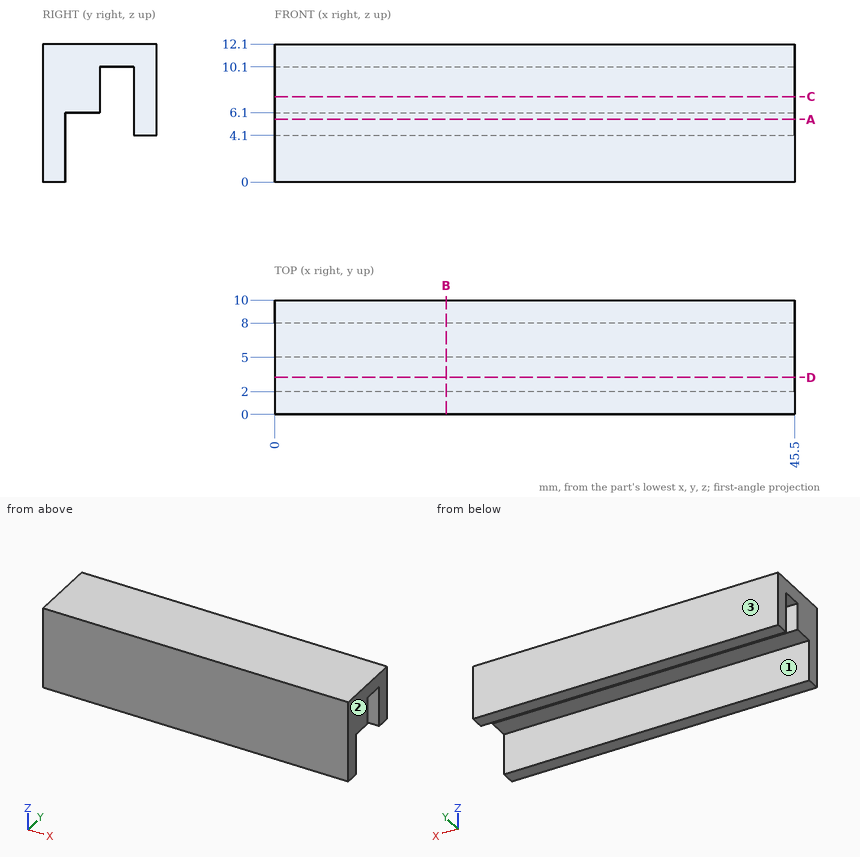
Geometry check sheet. Reference: drawing and pictorial views, mm from the part's lowest x, y, z. Coordinates: 2 decimals unless noted, no trailing zeros. Write each loop counter-clockwise with the first axis right and the second up, starting at its lowest first coordinate (ties: lowest second). Pieces come first, ordered by that corner, then holes. Notation, with made-up numbers: M -14,34.5 L 10,34.5 A14 ccw 10,59.5 Z; hole C 78.5,54.5 d6. An arc over 180 degrees is marked long. One line per question, with ' | ' between items.
1) Sectioned sample at A-A on z = 5.5. Record the cut outline in (x, y).
Solutions:
outline: M 0,0 L 45.5,0 L 45.5,2 L 0,2 Z; M 0,8 L 45.5,8 L 45.5,10 L 0,10 Z
2) Release check for a two-part mould opening along Y. For the marked faces 1, 2 and 3 record: +Y half, -Y half, draft (parallel to the pull), parting line (faces both ways), or undercut.
Solutions:
face 1: undercut | face 2: draft | face 3: +Y half
3) Sectioned sample at D-D on y = 3.25. Record the cut outline in (x, z), then the cut area to 3 significant figures.
Solutions:
outline: M 0,6.1 L 45.5,6.1 L 45.5,12.1 L 0,12.1 Z | area: 273 mm^2
4) Depth check by flat-ended pin: pin 1 Ø5 at (x, y) = (12.5, 7) entering from -Z; pin 2 Ø2 at (x, z) = (39, 2) entering from +Y; pin 3 Ø2.5 at (x, y) = (18.5, 6) entering from -Z. Enter the tip coordinate at first touch or a pass-through.
Solutions:
pin 1: z = 4.1 | pin 2: y = 2 | pin 3: z = 6.1
5) Sectioned sample at B-B on x = 15. Record the cut outline in (y, z).
Solutions:
outline: M 0,0 L 2,0 L 2,6.1 L 5,6.1 L 5,10.1 L 8,10.1 L 8,4.1 L 10,4.1 L 10,12.1 L 0,12.1 Z
6) Material ranges on L1, parallel to Y at x = 19, z = 8.5; L2, parallel to Y at x = 15, z = 6; L3, parallel to Z at x = 35.5, y = 3.25, recorded low to high.
Solutions:
L1: 0 to 5, 8 to 10 | L2: 0 to 2, 8 to 10 | L3: 6.1 to 12.1
7) Sectioned sample at C-C on z = 7.5. Record the cut outline in (x, y).
Solutions:
outline: M 0,0 L 45.5,0 L 45.5,5 L 0,5 Z; M 0,8 L 45.5,8 L 45.5,10 L 0,10 Z
